from build123d import *

# Parameters (mm, degrees)
ESQUISSE1_R             = 3
BASE_EXTRUSION_DEPTH    = 25
CHANFREIN2_SIZE         = 0.5
ESQUISSE2_W             = 2
ESQUISSE2_H             = 6
ENL_V_MAT_EXTRU_1_DEPTH = 6.5
ESQUISSE5_W             = 2
ESQUISSE5_H             = 6
ENL_V_MAT_EXTRU_3_DEPTH = 6.5
ESQUISSE4_R             = 1.2
ENL_V_MAT_EXTRU_2_DEPTH = 26.751893134
ENL_V_MAT_EXTRU_4_DEPTH = 3.5


with BuildPart() as part:
    # Esquisse1 → Base-Extrusion (new body)
    with BuildSketch(Plane.XY):
        with Locations(Location((0, 0, 0), (0, 0, 216.869897646))):
            Circle(ESQUISSE1_R)
    extrude(amount=BASE_EXTRUSION_DEPTH)

    # Chanfrein2
    chanfrein2_edges = [part.edges().sort_by_distance(p)[0] for p in [
        (2.4, 1.8, 0),
        (2.4, 1.8, 25),
    ]]
    chamfer(chanfrein2_edges, length=CHANFREIN2_SIZE)

    # Esquisse2 → Enlèv. mat.-Extru.1 (cut)
    with BuildSketch(Plane.XY.offset(25)):
        with Locations((3.4, 0)):
            Rectangle(ESQUISSE2_W, ESQUISSE2_H)
    extrude(amount=-ENL_V_MAT_EXTRU_1_DEPTH, mode=Mode.SUBTRACT)

    # Esquisse5 → Enlèv. mat.-Extru.3 (cut)
    with BuildSketch(Plane.XY.offset(25)):
        with Locations((-3.4, 0)):
            Rectangle(ESQUISSE5_W, ESQUISSE5_H)
    extrude(amount=-ENL_V_MAT_EXTRU_3_DEPTH, mode=Mode.SUBTRACT)

    # Esquisse4 → Enlèv. mat.-Extru.2 (cut, through all)
    with BuildSketch(Plane(origin=(2.4, 0, 0), x_dir=(0, 0, -1), z_dir=(1, 0, 0))):
        with Locations(Location((-22, 0, 0), (0, 0, 90))):
            Circle(ESQUISSE4_R)
    extrude(amount=-ENL_V_MAT_EXTRU_2_DEPTH, mode=Mode.SUBTRACT)

    # Esquisse6 → Enlèv. mat.-Extru.4 (cut)
    with BuildSketch(Plane(origin=(0, 0, 0), x_dir=(-1, 0, 0), z_dir=(0, 0, -1))):
        Polygon((-2, 0), (-0.999257658, 1.732479187), (0.999257658, 1.732479187), (2, 0), (0.999257658, -1.732479187), (-0.999257658, -1.732479187), align=None)
    extrude(amount=-ENL_V_MAT_EXTRU_4_DEPTH, mode=Mode.SUBTRACT)


solid = part.part
Geometry: final body of the model. Coordinates: model frame, mm. A direction names the side the tool comes from. Give positions to 0.01 mm unless a question says otherwise; leave off trailing zeros. Write each loop counter-clockwise with the first axis right and the second up, starting at its lowest first coordinate (ties: lowest second). Pieces come first, ordered by that corner, then holes. Notation, with made-up numbers: M 2.25,52 L 7.25,52 A21 cw 7.25,63 Z; hole C -25.75,41 d11. An arc over 180 degrees is marked long. Answer in a Markdown table with one row per item. Add a question column.
(1) Section B-B on x = 0. Return loops of the section in (y, z).
(2) Mould query, pull axis X, two halves, no side actions, for faces 1 (the flat face through (1.51, 0.85, 1.73)), 2 (the flat face through (-2.4, -1, 21)), 3 (the conical face through (-0.047, -2.635, 24.865)). Classes: +X half, -X half, draft (parallel to the pull), parting line (faces both ways), or undercut.
(3) Section C-C on z = 13.75. Return loops of the section in (x, y), and give its area (3 significant figures).
(4) Section D-D on z = 19. Return loops of the section in (x, y).
(5) First-contact query: pin 1 (3 mm diameter, centred on y = -0.5, z = 20.5, fed in from -X); pin 2 (2 mm diameter, centred on x = -1.5, z = 6, fed in from -Y); pin 3 (1.8 mm diameter, centred on y = 0.5, z = 22.5, fed in from +X). Flat tips, straight axial feed; report the tip coordinate or a pass-through.
(6) Section A-A on z = 22. Return loops of the section in (x, y), and give its area (3 significant figures).
(7) Reachability of faces 4 (the conical face through (0.047, 2.635, 24.865)), 5 (the flat face through (2.4, -1, 21)), 6 (the flat face through (0, -1.732, 2)) from +Z, -Z, +X, -X, +Y, -Y: full face, straight path, thin tool, end or side. Return the list, or none.
(8) Ray query, line 1 (Z direction, x = 0.55, y = 0); line 2 (Y direction, x = -0.1, z = 22.5); line 3 (Y direction, x = -0.1, z = 7.25). Return the intervals inside material, ascending.
Result set:
| question | item | result |
|---|---|---|
| 1 | outline | M -3,0.5 L -2.5,0 L -1.73,0 L -1.73,3.5 L 1.73,3.5 L 1.73,0 L 2.5,0 L 3,0.5 L 3,24.5 L 2.5,25 L -2.5,25 L -3,24.5 Z; hole C 0,22 d2.4 |
| 2 | face 1 | undercut |
| 2 | face 2 | -X half |
| 2 | face 3 | parting line |
| 3 | outline | C 0,0 d6 |
| 3 | area | 28.3 mm^2 |
| 4 | outline | M -2.4,-1.8 A3 ccw 2.4,-1.8 L 2.4,1.8 A3 ccw -2.4,1.8 Z |
| 5 | pin 1 | stops at x = -2.4 |
| 5 | pin 2 | stops at y = -2.96 |
| 5 | pin 3 | stops at x = 2.4 |
| 6 | outline | M -2.4,-1.8 A3 ccw 2.4,-1.8 L 2.4,-1.2 L -2.4,-1.2 Z; M -2.4,1.2 L 2.4,1.2 L 2.4,1.8 A3 ccw -2.4,1.8 Z |
| 6 | area | 13.8 mm^2 |
| 7 | face 4 | +Z, +Y |
| 7 | face 5 | +Z, +X, +Y, -Y |
| 7 | face 6 | -Z |
| 8 | line 1 | z = 3.5 to 20.8, 23.2 to 25 |
| 8 | line 2 | y = -3 to -1.09, 1.09 to 3 |
| 8 | line 3 | y = -3 to 3 |
